Check sheet for the modelled part. Datum: model origin and axes. Units: mm. A direction names the side the tool comes from. Give positions to 0.01 mm unless a question says otherwise; leave off trailing zeros. Order: outer loops, then holes, each group sorted by start corner. A loop starts at its lowest first (then second) coordinate and runs counter-clockwise, first axis right, second up.
Autodesk Fusion 360 part; units mm, degrees
sketch "Sketch1" plane through (0, 0, 0) normal (1, 0, 0) x (0, 1, 0)
  circle A0 centre (0, 0) radius 5
  dimension "d1" = 10
extrude "Extrude1" add sketch "Sketch1" along normal blind 130
sketch "Sketch2" plane through (130, 0, 0) normal (1, 0, 0) x (0, 0, -1)
  circle A0 centre (0, 0) radius 5
  circle A1 centre (0, 0) radius 4
  dimension "d4" = 8
extrude "Extrude2" cut sketch "Sketch2" against normal blind 50
sketch "Sketch3" plane through (0, 0, 0) normal (-1, 0, 0) x (0, 0, 1)
  circle A0 centre (0, 0) radius 5
  circle A1 centre (0, 0) radius 4
  dimension "d7" = 8
extrude "Extrude3" cut sketch "Sketch3" against normal blind 20
extrude "Extrude4" add 1 faces at (20, 4.6443, -0.348) along direction (-1, 0, 0) blind 5
extrude "Extrude5" cut 1 faces at (0, -0.5286, 1.4202) along direction (1, 0, 0) blind 5
extrude "Extrude6" add 1 faces at (80, 4.6443, 0.348) along direction (1, 0, 0) blind 52
extrude "Extrude7" add 1 faces at (130, -0.2204, 1.0288) along direction (1, 0, 0) blind 12
extrude "Extrude8" add 1 faces at (142, -0.2204, 1.0288) along direction (1, 0, 0) blind 40
sketch "Sketch4" plane through (0, 0, 0) normal (0, 1, 0) x (1, 0, 0)
sketch "Sketch5" plane through (0, 0, 0) normal (0, 1, 0) x (1, 0, 0)
sketch "Sketch6" plane through (0, 0, 0) normal (0, 1, 0) x (1, 0, 0)
  line L0 (132, 0) -> (107, 0)
  circle A0 centre (107, 0) radius 2.25
  dimension "d20" = 25
  dimension "d21" = 4.5
sketch "Sketch7" plane through (0, 0, 0) normal (0, 1, 0) x (1, 0, 0)
  line L0 (107, 0) -> (85, 0)
sketch "Sketch9" plane through (0, 0, 0) normal (0, 1, 0) x (1, 0, 0)
  circle A0 centre (102, 0) radius 2.25
  line L0 (132, -5) -> (132, 5)
  dimension "d32" = 4.5
  dimension "d33" = 30
extrude "Extrude13" cut sketch "Sketch9" along normal mid plane 20
sketch "Sketch10" plane through (0, 0, 0) normal (0, 1, 0) x (1, 0, 0)
extrude "Extrude14" add 1 faces at (5, -0.5286, 1.4202) along direction (-1, 0, 0) blind 63
extrude "Extrude15" add 1 faces at (15, 4.6443, -0.348) along direction (-1, 0, 0) blind 63
sketch "Sketch8" plane through (0, 0, 0) normal (0, 1, 0) x (1, 0, 0)
extrude "Extrude11" [suppressed]
extrude "Extrude12" [suppressed]
1) Depth check by flat-ended pin: pin 1 Ø1 at (x, z) = (-16.5, 2) entering from +Y; pin 2 Ø3 at (x, y) = (2.5, 3.5) entering from -Z; pin 3 Ø1 at (x, z) = (52, -3.5) entering from -Y. Enter the tip coordinate at first touch or a pass-through.
Recorded:
pin 1: stops at y = 4.77
pin 2: stops at z = -4.58
pin 3: stops at y = -4
2) Draft check along Z on faces 1 (the face through (-58, 0, 0)), 2 (the face through (43.26, -1.08, -4.88)), 3 (the face through (104.08, -0.07, -0.86)). Enter one of: +Z half, -Z half, draft (parallel to the pull), parting line (faces both ways), or undercut.
Recorded:
face 1: draft
face 2: parting line
face 3: undercut
3) Material ranges on L1, parallel to X at y = -0.75, z = 0; L2, parallel to Z at x = 102, y = 0; L3, parallel to Z at x = 19, y = -0.5, recorded low to high.
Recorded:
L1: x = -58 to 99.75, 104.25 to 182
L2: z = -5 to -2.25, 2.25 to 5
L3: z = -4.97 to 4.97
4) Section check C-C, the plane x = -19.5. Record the cut outline in (y, z).
Recorded:
outline: circle Ø10 at (0, 0)
5) Section check A-A, the plane z = 0. Record the cut outline in (x, y), then the cut area to 4 significant figures.
Recorded:
outline: (-58, -4) - (-48, -4) - (-48, -5) - (99.75, -5) - (99.75, 5) - (-48, 5) - (-48, 4) - (-58, 4) - close; (104.25, -5) - (132, -5) - (132, -4) - (182, -4) - (182, 4) - (132, 4) - (132, 5) - (104.25, 5) - close
area: 2,235 mm2
6) Set-up check for faces 4 (the face through (-52.93, 3.905, -0.867)), 5 (the face through (156.65, 3.905, 0.867)), 6 (the face through (182, 0, 0)): record each of +Z, -Z, +X, -X, +Y, -Y from which the full face is reachable in a straight line by a thin tool's end or side.
Recorded:
face 4: -X
face 5: +X
face 6: +Z, -Z, +X, +Y, -Y
7) Section check B-B, the plane y = 0. Record the cut outline in (x, z), then the cut area to 3 significant figures.
Recorded:
outline: (-58, -4) - (-48, -4) - (-48, -5) - (132, -5) - (132, -4) - (182, -4) - (182, 4) - (132, 4) - (132, 5) - (-48, 5) - (-48, 4) - (-58, 4) - close; hole circle Ø4.5 at (102, 0)
area: 2,260 mm2
